Work out the finished part from the listing and answer in its coordinate system (mm). Coordinates: 2 decimals unless noted, no trailing zeros. Order: outer loops, then holes, each group sorted by start corner. A loop starts at its lowest first (then second) coordinate and runs counter-clockwise, first axis right, second up. Notation, with made-up numbers: M 1,49 L 16,49 A17 ccw 16,81 Z; hole C -21,-25.75 d6. An arc over 180 degrees is marked long. Use a Markdown table: item, result.
from build123d import *

# Parameters (mm, degrees)
SKETCH1_R            = 2.0828
BOSS_EXTRUDE1_DEPTH  = 3.175
M3_CLEARANCE_HOLE1_D = 3.2
SKETCH5_W            = 19.8
SKETCH5_H            = 4.5
CUT_EXTRUDE1_DEPTH   = 265.974627323
SKETCH7_R            = 2.413
CUT_EXTRUDE2_DEPTH   = 265.974627323


with BuildPart() as part:
    # Sketch1 → Boss-Extrude1 (new body)
    with BuildSketch(Plane(origin=(0, 0, 0), x_dir=(1, 0, 0), z_dir=(0, 1, 0))):
        Polygon((28.855389821, 184.15), (123.544610179, 184.15), (176.5, 131.194610179), (182.5, 125.194610179), (190.5, 117.194610179), (190.5, 22.505389821), (182.5, 14.505389821), (176.5, 8.505389821), (137.544610179, -30.45), (131.544610179, -36.45), (123.544610179, -44.45), (28.855389821, -44.45), (20.855389821, -36.45), (14.855389821, -30.45), (-24.1, 8.505389821), (-30.1, 14.505389821), (-38.1, 22.505389821), (-38.1, 117.194610179), (-30.1, 125.194610179), (-24.1, 131.194610179), align=None)
        with Locations(Location((24.384, 12.7, 0), (0, 0, 270))):
            Circle(SKETCH1_R, mode=Mode.SUBTRACT)
        with Locations(Location((128.016, 12.7, 0), (0, 0, 90))):
            Circle(SKETCH1_R, mode=Mode.SUBTRACT)
        with Locations(Location((128.016, 127, 0), (0, 0, 270))):
            Circle(SKETCH1_R, mode=Mode.SUBTRACT)
        with Locations(Location((24.384, 127, 0), (0, 0, 90))):
            Circle(SKETCH1_R, mode=Mode.SUBTRACT)
    extrude(amount=BOSS_EXTRUDE1_DEPTH)

    # M3 Clearance Hole1 (through all)
    with Locations(Plane(origin=(0, 3.175, 0), x_dir=(1, 0, 0), z_dir=(0, 1, 0))):
        with Locations((-31.5214, 106.313101446), (-31.5214, 91.073101446), (-31.5214, 55.8795536), (-31.5214, 40.6395536), (-31.5214, 25.230335162), (-16.2814, 25.230335162), (68.58, -37.8714), (83.82, -37.8714), (183.9214, 25.230335162), (168.6814, 25.230335162), (183.9214, 40.6395536), (183.9214, 55.8795536), (183.9214, 91.073101446), (183.9214, 106.313101446)):
            Hole(M3_CLEARANCE_HOLE1_D / 2)

    # Sketch5 → Cut-Extrude1 (cut, through all)
    with BuildSketch(Plane(origin=(0, 3.175, 0), x_dir=(1, 0, 0), z_dir=(0, 1, 0))):
        with Locations((76.2, 67.6)):
            Rectangle(SKETCH5_W, SKETCH5_H)
    extrude(amount=-CUT_EXTRUDE1_DEPTH, mode=Mode.SUBTRACT)

    # Sketch7 → Cut-Extrude2 (cut, through all)
    with BuildSketch(Plane(origin=(0, 3.175, 0), x_dir=(1, 0, 0), z_dir=(0, 1, 0))):
        with Locations(Location((50.8, 154.263560488, 0), (0, 0, 270))):
            Circle(SKETCH7_R)
        with Locations(Location((101.6, 154.263560488, 0), (0, 0, 90))):
            Circle(SKETCH7_R)
    extrude(amount=-CUT_EXTRUDE2_DEPTH, mode=Mode.SUBTRACT)


solid = part.part
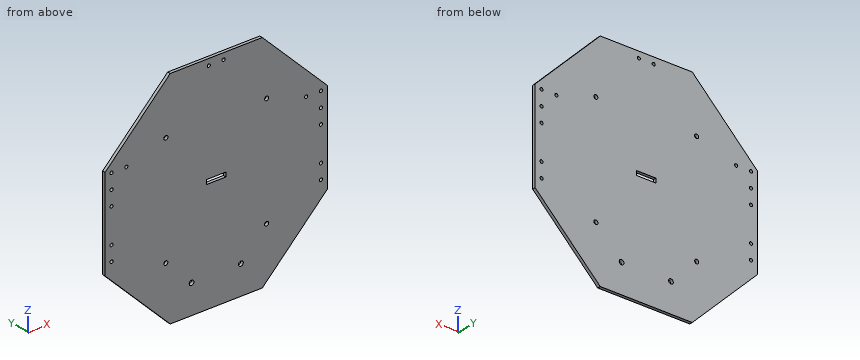
(1) A cutting plane is placed at A-A (y = 1.4). Give the number of separate pieces and of enclosed holes in the cut face, then the cut area to 3 significant figures.
Conclusion:
| item | result |
|---|---|
| separate pieces | 1 |
| enclosed holes | 21 |
| area | 43,000 mm2 |
(2) A cutting plane is placed at C-C (z = -166). Determine the outline of the cut face in (x, y) (3 decimals), then the cut area to 3 significant figures.
Conclusion:
| item | result |
|---|---|
| outline | M 10.705,0 L 141.695,0 L 141.695,3.175 L 10.705,3.175 Z |
| area | 416 mm2 |
(3) Straight lines are drawn through the part: L1, parallel to X at y = 0.25, z = -69; L2, parallel to Z at x = 101.6, y = 1.05; L3, parallel to X at y = 1.85, z = -127. For each, find the intervals that lie inside material, in ascending order.
Conclusion:
| item | result |
|---|---|
| L1 | -38.1 to 66.3, 86.1 to 190.5 |
| L2 | -184.15 to -156.68, -151.85 to 44.45 |
| L3 | -28.29 to 22.3, 26.47 to 125.93, 130.1 to 180.69 |
(4) A cutting plane is placed at B-B (x = 153). Determine the outline of the cut face in (y, z) (3 decimals), then the cut area to 3 significant figures.
Conclusion:
| item | result |
|---|---|
| outline | M 0,-154.695 L 3.175,-154.695 L 3.175,14.995 L 0,14.995 Z |
| area | 539 mm2 |
